from build123d import *

# Parameters (mm, degrees)
F0_R      = 9.5
F1_DEPTH  = 84
F3_DEPTH  = 12.5
F5_DEPTH  = 12.5
F7_W      = 4
F7_H      = 3.791283
F8_DEPTH  = 50.14
F10_DEPTH = 39.6
F12_DEPTH = 12.5


with BuildPart() as f1:
    # F0 (on Front) → F1 (new body, symmetric)
    with BuildSketch(Plane.XZ):
        with BuildLine():
            Line((-11.895642, 3.839754), (-11.895642, -3.839754))
            ThreePointArc((-11.895642, -3.839754), (-11.548494, -4.783543), (-11.126605, -5.696373))
            Line((-11.126605, -5.696373), (-5.696373, -11.126605))
            ThreePointArc((-5.696373, -11.126605), (-4.783543, -11.548494), (-3.839754, -11.895642))
            Line((-3.839754, -11.895642), (3.839754, -11.895642))
            ThreePointArc((3.839754, -11.895642), (4.783543, -11.548494), (5.696373, -11.126605))
            Line((5.696373, -11.126605), (11.126605, -5.696373))
            ThreePointArc((11.126605, -5.696373), (11.548494, -4.783543), (11.895642, -3.839754))
            Line((11.895642, -3.839754), (11.895642, 3.839754))
            ThreePointArc((11.895642, 3.839754), (11.548494, 4.783543), (11.126605, 5.696373))
            Line((11.126605, 5.696373), (5.696373, 11.126605))
            ThreePointArc((5.696373, 11.126605), (4.783543, 11.548494), (3.839754, 11.895642))
            Line((3.839754, 11.895642), (-3.839754, 11.895642))
            ThreePointArc((-3.839754, 11.895642), (-4.783543, 11.548494), (-5.696373, 11.126605))
            Line((-5.696373, 11.126605), (-11.126605, 5.696373))
            ThreePointArc((-11.126605, 5.696373), (-11.548494, 4.783543), (-11.895642, 3.839754))
        make_face()
        Circle(F0_R, mode=Mode.SUBTRACT)
    extrude(amount=F1_DEPTH, both=True)

    # F2 (on Right) → F3 (cut, symmetric)
    with BuildSketch(Plane.YZ):
        with BuildLine():
            Line((-1, 23.303589), (-54, 23.303589))
            Line((-54, 23.303589), (-54, 10.395642))
            ThreePointArc((-54, 10.395642), (-52.535534, 6.860108), (-49, 5.395642))
            Line((-49, 5.395642), (-6, 5.395642))
            ThreePointArc((-6, 5.395642), (-2.464466, 6.860108), (-1, 10.395642))
            Line((-1, 10.395642), (-1, 23.303589))
        make_face()
    extrude(amount=F3_DEPTH, both=True, mode=Mode.SUBTRACT)

    # F4 (on Right) → F5 (cut, symmetric)
    with BuildSketch(Plane.YZ):
        Polygon((-44.4, -6.895642), (-44.4, -11.895642), (-44.4, -23.509938), (-3, -23.509938), (-3, -6.895642), align=None)
    extrude(amount=F5_DEPTH, both=True, mode=Mode.SUBTRACT)

    # F7 (on offset) → F8 (cut)
    with BuildSketch(Plane.XZ.offset(84)):
        with Locations((0, -11.895641)):
            Rectangle(F7_W, F7_H)
    extrude(amount=-F8_DEPTH, mode=Mode.SUBTRACT)

    # F9 (on offset) → F10 (join, through all)
    with BuildSketch(Plane.XZ.offset(84)):
        with BuildLine():
            Line((-2, -11.895642), (-3.839754, -11.895642))
            ThreePointArc((-3.839754, -11.895642), (-2.928278, -12.152168), (-2, -12.338963))
            Line((-2, -12.338963), (-2, -11.895642))
        make_face()
        with BuildLine():
            Line((3.839754, -11.895642), (2, -11.895642))
            Line((2, -11.895642), (2, -12.338963))
            ThreePointArc((2, -12.338963), (2.928278, -12.152168), (3.839754, -11.895642))
        make_face()
    extrude(amount=-F10_DEPTH)

    # F11 (on Right) → F12 (cut, symmetric)
    with BuildSketch(Plane.YZ):
        Polygon((-84, -9.838963), (-84, -12.338963), (-81.5, -12.338963), align=None)
    extrude(amount=F12_DEPTH, both=True, mode=Mode.SUBTRACT)

    # F13 (on Right) → F14 (revolve, cut)
    with BuildSketch(Plane.YZ):
        Polygon((-86.791411, -19.086694), (-67.18528, -15.093563), (-84, -10.338963), align=None)
    revolve(axis=Axis((0, -51.056053, 0), (0, -1, 0)), mode=Mode.SUBTRACT)


solid = f1.part
Can you work these out from the model? Positions are in its coordinate system, mm. A direction names the side the tool comes from. Coordinates: 2 decimals unless noted, no trailing zeros. Write each loop counter-clockwise with the first axis right and the second up, starting at its lowest first coordinate (ties: lowest second). Pieces come first, ordered by that corner, then holes. Notation, with made-up numbers: (35, -3) -> (84, -3) arc R26 ccw to (84, 33) -> close; hole circle Ø3 at (81.25, -39). An arc over 180 degrees is marked (long way). Write each question's results on one line, items separated by ' | '. Start each with the question number.
Item 1: I'm going to push flat-ended pins straight in: P1, Ø3.5, axis at x = -8, y = -29, coming from the -Z side; P2, Ø1.7, axis at x = -10, y = -36.5, coming from the +Z side; P3, Ø8.5, axis at x = 0, y = 22.5, coming from the -Z side. Where does each tip first touch, or does it pass through?
Item 2: On a 3-axis mill with a long thin cutter (end or side, diameter ignored), from which of +Z, -Z, +X, -X, +Y, -Y can I reach the whole of each face in a straight line? I mean faces 5 (the flat face through (0, -3, -10)), 6 (the flat face through (0, 40, -11.896)), 7 (the cylindrical face through (-0.783, -1.055, 9.653)), 8 (the flat face through (0, -66, 11.896)), 9 (the flat face through (0, -64, -10)). Say none if no direction works.
Item 3: Please list where these lines run through material, in increasing order: probe 1 along Z at (x, y) = (0, 14); probe 2 along X at (y, z) = (-66, -3); probe 3 along Z at (x, y) = (-8.5, -44.5).
Item 4: If we section it at A-A, the plane y = 73: Write out the boundary of the cut face in (x, z).
Item 5: If we section it at C-C, the plane x = 0: Write out the boundary of the cut face in (y, z), and give its area (3 significant figures).
Item 6: Thinking about a two-plate mould opening in X: for faces 1 (the flat face through (-8, -23, -6.896)), 2 (the flat face through (8.45, -64.796, 8.373)), 3 (the conical face through (-9.72, -83.63, -3.82)), 4 (the cylindrical face through (-2.059, 1.176, -9.274)), which applies, released by +X, released by -X, zero draft, split by the parting line, or undercut?
Item 7: If we section it at B-B, the plane z = 0: Write out the boundary of the cut face in (x, y), and give its area (3 significant figures).
Answer block:
1) P1: z = -6.9 | P2: z = 5.4 | P3: z = -11.9
2) face 5: -Z, +X, -X | face 6: -Z, +X, -X, +Y | face 7: +Z, +X, -X | face 8: +Z, +X, -X, +Y, -Y | face 9: -Z, -Y
3) probe 1: -11.9 to -9.5, 9.5 to 11.9 | probe 2: -11.9 to -9.01, 9.01 to 11.9 | probe 3: -8.32 to -4.24, 4.24 to 5.4
4) outline: (-11.9, -3.84) arc R12.5 ccw to (-11.13, -5.7) -> (-5.7, -11.13) arc R12.5 ccw to (-3.84, -11.9) -> (3.84, -11.9) arc R12.5 ccw to (5.7, -11.13) -> (11.13, -5.7) arc R12.5 ccw to (11.9, -3.84) -> (11.9, 3.84) arc R12.5 ccw to (11.13, 5.7) -> (5.7, 11.13) arc R12.5 ccw to (3.84, 11.9) -> (-3.84, 11.9) arc R12.5 ccw to (-5.7, 11.13) -> (-11.13, 5.7) arc R12.5 ccw to (-11.9, 3.84) -> close; hole circle Ø19 at (0, 0)
5) outline: (-84, -9.84) -> (-83.84, -10) -> (-44.4, -10) -> (-44.4, -9.5) -> (-84, -9.5) -> close; (-84, 9.5) -> (-53.92, 9.5) arc R5 cw to (-54, 10.4) -> (-54, 11.9) -> (-78.49, 11.9) -> (-84, 10.34) -> close; (-3, -11.9) -> (84, -11.9) -> (84, -9.5) -> (-3, -9.5) -> close; (-1.08, 9.5) -> (84, 9.5) -> (84, 11.9) -> (-1, 11.9) -> (-1, 10.4) arc R5 cw to start | area: 499 mm²
6) face 1: zero draft | face 2: released by +X | face 3: split by the parting line | face 4: undercut
7) outline: (-11.9, -78.49) -> (-10.34, -84) -> (-9.5, -84) -> (-9.5, 84) -> (-11.9, 84) -> close; (9.5, -84) -> (10.34, -84) -> (11.9, -78.49) -> (11.9, 84) -> (9.5, 84) -> close | area: 796 mm²
